Geometry check sheet. Reference: the model listing, model coordinates, mm. A direction names the side the tool comes from. Round coordinates to 2 decimals unless told otherwise and drop trailing zeros. Write each loop counter-clockwise with the first axis right and the second up, starting at its lowest first coordinate (ties: lowest second). Pieces come first, ordered by that corner, then holes. Notation, with made-up numbers: (-2.5, 19) -> (35.5, 19) arc R32 cw to (35.5, 48) -> close; hole circle Ø3 at (-5, -14). An arc over 180 degrees is marked (long way). Return JSON: item names as keys, results as strings. Group by question number.
from build123d import *

# Parameters (mm, degrees)
SKETCH_1_R      = 5.05
SKETCH_1_R_2    = 2.05
SKETCH_1_R_3    = 3.783876232
EXTRUDE_1_DEPTH = 2


with BuildPart() as part:
    # 草图1 → 凸台-拉伸1 (new body)
    with BuildSketch(Plane.XY):
        with BuildLine():
            Line((-5.587732913, 20.736278596), (-5.587732913, 24.736278596))
            Line((-5.587732913, 24.736278596), (-4.137732913, 24.736278596))
            Line((-4.137732913, 24.736278596), (-4.137732913, 27.936278596))
            Line((-4.137732913, 27.936278596), (-5.587732913, 27.936278596))
            Line((-5.587732913, 27.936278596), (-5.587732913, 31.136278596))
            Line((-5.587732913, 31.136278596), (-9.687732913, 31.136278596))
            Line((-9.687732913, 31.136278596), (-9.687732913, 27.936278596))
            Line((-9.687732913, 27.936278596), (-11.137732913, 27.936278596))
            Line((-11.137732913, 27.936278596), (-11.137732913, 24.736278596))
            Line((-11.137732913, 24.736278596), (-9.687732913, 24.736278596))
            Line((-9.687732913, 24.736278596), (-9.687732913, 20.736278596))
            Line((-9.687732913, 20.736278596), (-18.637732913, 20.736278596))
            Line((-18.637732913, 20.736278596), (-18.637732913, 14.736278596))
            Line((-18.637732913, 14.736278596), (-26.637732913, 14.736278596))
            Line((-26.637732913, 14.736278596), (-26.637732913, 20.736278596))
            Line((-26.637732913, 20.736278596), (-30.637732913, 20.736278596))
            Line((-30.637732913, 20.736278596), (-30.637732913, 42.62233047))
            Line((-30.637732913, 42.62233047), (-27.637732913, 70.736278596))
            ThreePointArc((-27.637732913, 70.736278596), (-7.637732913, 90.736278596), (12.362267087, 70.736278596))
            Line((12.362267087, 70.736278596), (15.362267087, 42.62233047))
            Line((15.362267087, 42.62233047), (15.362267087, 20.736278596))
            Line((15.362267087, 20.736278596), (11.362267087, 20.736278596))
            Line((11.362267087, 20.736278596), (11.362267087, 14.736278596))
            Line((11.362267087, 14.736278596), (3.362267087, 14.736278596))
            Line((3.362267087, 14.736278596), (3.362267087, 20.736278596))
            Line((3.362267087, 20.736278596), (-5.587732913, 20.736278596))
        make_face()
        with Locations((-7.637732913, 70.736278596)):
            Circle(SKETCH_1_R, mode=Mode.SUBTRACT)
        with Locations((10.039936617, 53.058609066)):
            Circle(SKETCH_1_R_2, mode=Mode.SUBTRACT)
        with Locations(Location((-25.315402443, 53.058609066, 0), (0, 0, 180))):
            Circle(SKETCH_1_R_2, mode=Mode.SUBTRACT)
        with Locations((-7.637732913, 38.004477847)):
            Circle(SKETCH_1_R_3, mode=Mode.SUBTRACT)
    extrude(amount=EXTRUDE_1_DEPTH)


solid = part.part
1) Material ranges on probe 1 along Y at (x, z) = (-8, 1.3); probe 2 along X at (y, z) = (25, 0.9); probe 3 along Y at (x, z) = (-6.5, 0.25), recorded low to high. Write a range as [from, to].
2) Sectioned sample at B-B on y = 68.5. Enter the section's corners in (x, z).
3) Sectioned sample at C-C on y = 52. Enter the section's corners in (x, z), and give its area (3 significant figures).
4) Sectioned sample at D-D on x = -16.5. Enter the section's corners in (y, z), and give its area (3 significant figures).
5) Tool access check on faces 5 (the face through (-5.588, 23, 1)), 6 (the face through (-26.638, 18, 1)), 7 (the face through (-10, 24.736, 1)). Record the directions out of +Z, -Z, +X, -X, +Y, -Y that give a thin tool (end or side, any length) a straight path to the whole face; none if there is none.
6) Mould release check, pull along Y, two halves, no side actions. Record for faces 1 (the face through (-29, 20.736, 1)), 2 (the face through (-4.138, 26, 1)), 3 (the face through (-26.42, 51.33, 0.99)), 4 (the face through (13.84, 56.88, 0.99)): +Y half, -Y half, draft (parallel to the pull), parting line (faces both ways), or undercut.
7) Go/stop test with flat-tipped pins: P1, Ø0.6, axis at y = 18.5, z = 1, coming from the +X side; P2, Ø0.6, axis at x = 13.5, z = 1, coming from the -Y side; P3, Ø1, axis at x = -18.5, z = 0.5, coming from the +Y side. Record where each tip stops, or that it passes through.
8) Sectioned sample at A-A on z = 1.1. State how many separate pieces and enclosed holes the cut face has, and give its area (3 significant figures).
Evaluation:
{
 "1": {"probe 1": "y = [31.14, 34.24], [41.77, 65.7], [75.77, 90.73]", "probe 2": "x = [-30.64, -11.14], [-4.14, 15.36]", "probe 3": "y = [31.14, 34.4], [41.61, 65.82], [75.66, 90.7]"},
 "2": {"outline": "(-27.88, 0) -> (-12.17, 0) -> (-12.17, 2) -> (-27.88, 2) -> close; (-3.11, 0) -> (12.6, 0) -> (12.6, 2) -> (-3.11, 2) -> close"},
 "3": {"outline": "(-29.64, 0) -> (-27.07, 0) -> (-27.07, 2) -> (-29.64, 2) -> close; (-23.56, 0) -> (8.28, 0) -> (8.28, 2) -> (-23.56, 2) -> close; (11.8, 0) -> (14.36, 0) -> (14.36, 2) -> (11.8, 2) -> close", "area": "74.0 mm2"},
 "4": {"outline": "(20.74, 0) -> (88.67, 0) -> (88.67, 2) -> (20.74, 2) -> close", "area": "136 mm2"},
 "5": {"face 5": "+Z, -Z, -Y", "face 6": "+Z, -Z, -X, -Y", "face 7": "+Z, -Z"},
 "6": {"face 1": "-Y half", "face 2": "undercut", "face 3": "undercut", "face 4": "+Y half"},
 "7": {"P1": "stops at x = 11.36", "P2": "stops at y = 20.74", "P3": "stops at y = 87.84"},
 "8": {"separate pieces": "1", "enclosed holes": "4", "area": "2,740 mm2"}
}
